Check sheet for the modelled part. Datum: model origin and axes. Units: mm. Give positions to 0.01 mm unless a question says otherwise; leave off trailing zeros. Order: outer loops, then holes, each group sorted by start corner. A loop starts at its lowest first (then second) coordinate and runs counter-clockwise, first axis right, second up. Notation, with made-up numbers: (-19.5, -33) -> (21.5, -33) arc R18 cw to (21.5, 1) -> close; hole circle Ø5 at (-1.5, 0.25). An arc over 180 degrees is marked (long way). Answer in a Markdown table with one row per item. Add a question column.
(1) Cross-section at A-A (y = 20.25). Record the cut outline in (x, z).
(2) Cross-section at D-D (x = -22). Record the cut outline in (y, z).
(3) Cross-section at B-B (z = 2.7). Record the cut outline in (x, y), then the cut area to 4 significant figures.
(4) Cross-section at C-C (y = -1.25). Record the cut outline in (x, z).
(5) Thickness scan on L1, parallel to X at y = 20.75, z = 4.2; L2, parallel to X at y = -3.5, z = 0.55; L3, parallel to Y at x = -29, z = 2. Record the ranges inside material, lowest first. Write a range as [from, to].
(6) Go/stop test with flat-tipped pins: pin 1 (2.5 mm diameter, centred on x = -46.5, z = 2, fed in from -Y); pin 2 (2.5 mm diameter, centred on x = -39, z = 1.5, fed in from +Y). Record where each tip stops, or that it passes through.
```python
from build123d import *

# Parameters (mm, degrees)
SKETCH1_W           = 10
SKETCH1_H           = 5
SKETCH1_W_2         = 25
SKETCH1_W_3         = 20
BOSS_EXTRUDE1_DEPTH = 5
SKETCH2_W           = 5
SKETCH2_H           = 5
CUT_EXTRUDE1_DEPTH  = 1


with BuildPart() as part:
    # Sketch1 → Boss-Extrude1 (new body)
    with BuildSketch(Plane.XY):
        Polygon((-20, 0), (0, 0), (0, 17.5), (-20, 17.5), (-65, 17.5), (-75, 17.5), (-80, 17.5), (-90, 17.5), (-90, 0), (-65, 0), align=None)
        with Locations((-85, 20)):
            Rectangle(SKETCH1_W, SKETCH1_H)
        with Locations((-70, 20)):
            Rectangle(SKETCH1_W, SKETCH1_H)
        with Locations((-77.5, -2.5)):
            Rectangle(SKETCH1_W_2, SKETCH1_H)
        with Locations((-10, -2.5)):
            Rectangle(SKETCH1_W_3, SKETCH1_H)
        with Locations((-10, 20)):
            Rectangle(SKETCH1_W_3, SKETCH1_H)
    extrude(amount=BOSS_EXTRUDE1_DEPTH)

    # Sketch2 → Cut-Extrude1 (cut)
    with BuildSketch(Plane(origin=(-65, 0, 0), x_dir=(0, 0, -1), z_dir=(1, 0, 0))):
        with Locations((-2.5, 20)):
            Rectangle(SKETCH2_W, SKETCH2_H)
    extrude(amount=-CUT_EXTRUDE1_DEPTH, mode=Mode.SUBTRACT)


solid = part.part
```
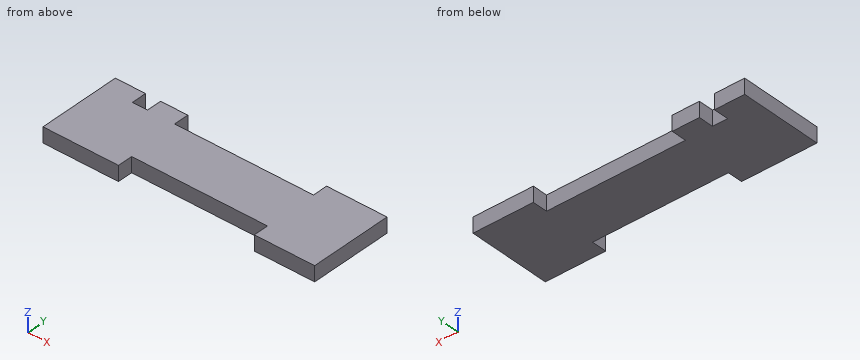
Answer below:
| question | item | result |
|---|---|---|
| 1 | outline | (-90, 0) -> (-80, 0) -> (-80, 5) -> (-90, 5) -> close; (-75, 0) -> (-66, 0) -> (-66, 5) -> (-75, 5) -> close; (-20, 0) -> (0, 0) -> (0, 5) -> (-20, 5) -> close |
| 2 | outline | (0, 0) -> (17.5, 0) -> (17.5, 5) -> (0, 5) -> close |
| 3 | outline | (-90, -5) -> (-65, -5) -> (-65, 0) -> (-20, 0) -> (-20, -5) -> (0, -5) -> (0, 22.5) -> (-20, 22.5) -> (-20, 17.5) -> (-66, 17.5) -> (-66, 22.5) -> (-75, 22.5) -> (-75, 17.5) -> (-80, 17.5) -> (-80, 22.5) -> (-90, 22.5) -> close |
| 3 | area | 1,995 mm² |
| 4 | outline | (-90, 0) -> (-65, 0) -> (-65, 5) -> (-90, 5) -> close; (-20, 0) -> (0, 0) -> (0, 5) -> (-20, 5) -> close |
| 5 | L1 | x = [-90, -80], [-75, -66], [-20, 0] |
| 5 | L2 | x = [-90, -65], [-20, 0] |
| 5 | L3 | y = [0, 17.5] |
| 6 | pin 1 | stops at y = 0 |
| 6 | pin 2 | stops at y = 17.5 |
